from build123d import *

# Parameters (mm, degrees)
SKETCH1_R                = 152
BOSS_EXTRUDE1_DEPTH      = 3
SKETCH2_R                = 12.5
CUT_EXTRUDE1_DEPTH       = 3
SKETCH3_R                = 20
BOSS_EXTRUDE2_DEPTH      = 0.1
BOSS_EXTRUDE2_DEPTH_BACK = 3.2
SKETCH4_R                = 12.5
CUT_EXTRUDE2_DEPTH       = 50.1


with BuildPart() as part:
    # Sketch1 → Boss-Extrude1 (new body)
    with BuildSketch(Plane.XY):
        Circle(SKETCH1_R)
    extrude(amount=BOSS_EXTRUDE1_DEPTH)

    # Sketch2 → Cut-Extrude1 (cut)
    with BuildSketch(Plane.XY.offset(3)):
        Circle(SKETCH2_R)
    extrude(amount=-CUT_EXTRUDE1_DEPTH, mode=Mode.SUBTRACT)

    # Sketch3 → Boss-Extrude2 (add, two sides)
    with BuildSketch(Plane.XY.offset(3)) as boss_extrude2_sk:
        Circle(SKETCH3_R)
    extrude(amount=BOSS_EXTRUDE2_DEPTH)
    extrude(boss_extrude2_sk.sketch, amount=-BOSS_EXTRUDE2_DEPTH_BACK)

    # Sketch4 → Cut-Extrude2 (cut)
    with BuildSketch(Plane(origin=(0, 0, -0.2), x_dir=(-1, 0, 0), z_dir=(0, 0, -1))):
        Circle(SKETCH4_R)
    extrude(amount=-CUT_EXTRUDE2_DEPTH, mode=Mode.SUBTRACT)


solid = part.part
Can you work these out from the model? Positions are in its coordinate system, mm. Give positions to 0.01 mm unless a question says otherwise; leave off trailing zeros. Order: outer loops, then holes, each group sorted by start corner. A loop starts at its lowest first (then second) coordinate and runs counter-clockwise, first axis right, second up. Notation, with made-up numbers: M -35,-28.75 L 14,-28.75 A18 ccw 14,-23.75 Z; hole C 27.25,44 d3. An arc over 180 degrees is marked long. One line per item, written item: value.
Item 1: If we section it at C-C on z = 1.7: Write out the boundary of the cut face in (x, y), and give its area (3 significant figures).
Verdict:
outline: C 0,0 d304; hole C 0,0 d25
area: 72,100 mm2
Item 2: If we section it at A-A on x = 0: Write out the boundary of the cut face in (y, z).
Verdict:
outline: M -152,0 L -20,0 L -20,-0.2 L -12.5,-0.2 L -12.5,3.1 L -20,3.1 L -20,3 L -152,3 Z; M 12.5,-0.2 L 20,-0.2 L 20,0 L 152,0 L 152,3 L 20,3 L 20,3.1 L 12.5,3.1 Z
Item 3: Please list where these lines run through material, in increasing order: line 1 (Y direction, x = 0, z = 1.15); line 2 (Z direction, x = -10, y = 104); line 3 (X direction, y = 41, z = 1.85).
Verdict:
line 1: -152 to -12.5, 12.5 to 152
line 2: 0 to 3
line 3: -146.37 to 146.37
Item 4: If we section it at D-D on y = -38: Write out the boundary of the cut face in (x, z), and give its area (3 significant figures).
Verdict:
outline: M -147.17,0 L 147.17,0 L 147.17,3 L -147.17,3 Z
area: 883 mm2
Item 5: For pin 1 (15 mm diameter, centred on x = 0, y = 0, fed in from -Z); pin 2 (1 mm diameter, centred on y = 74, z = 1, fed in from -X); pin 3 (2 mm diameter, centred on x = 32.5, y = -113.5, fed in from -Z); pin 4 (1.5 mm diameter, centred on x = -15.5, z = 2, fed in from -Y), each with a flat end and sliding along its axis, tell me the tip position at first contact or that it passes through.
Verdict:
pin 1: through
pin 2: x = -133.05
pin 3: z = 0
pin 4: y = -151.28
